Can you work these out from the model? Positions are in its coordinate system, mm. A direction names the side the tool comes from. Round coordinates to 2 decimals unless told otherwise and drop trailing zeros. Write each loop counter-clockwise with the first axis right and the second up, starting at its lowest first coordinate (ties: lowest second). Pieces come first, ordered by that corner, then holes. Notation, with made-up numbers: (40.25, 74) -> (47.25, 74) arc R15 ccw to (47.25, 100) -> close; hole circle Ø8 at (89.25, 35.25). An arc over 180 degrees is marked (long way). Use CSV: the item, a comma, the result in double quotes.
```python
from build123d import *

# Parameters (mm, degrees)
SKETCH1_W                = 29.718
SKETCH1_H                = 10.668
BOSS_EXTRUDE1_DEPTH      = 10.16
SKETCH2_W                = 10.668
SKETCH2_H                = 10.668
CUT_EXTRUDE1_DEPTH       = 7.62
M6_CLEARANCE_HOLE1_D     = 6.8032
M6_CLEARANCE_HOLE1_DEPTH = 32.4993
M6_CLEARANCE_HOLE1_TIP   = 2.043887482


with BuildPart() as part:
    # Sketch1 → Boss-Extrude1 (new body)
    with BuildSketch(Plane(origin=(0, 0, 0), x_dir=(1, 0, 0), z_dir=(0, 1, 0))):
        Rectangle(SKETCH1_W, SKETCH1_H)
    extrude(amount=BOSS_EXTRUDE1_DEPTH)

    # Sketch2 → Cut-Extrude1 (cut)
    with BuildSketch(Plane(origin=(0, 0, 0), x_dir=(-1, 0, 0), z_dir=(0, -1, 0))):
        with Locations((-9.525, 0)):
            Rectangle(SKETCH2_W, SKETCH2_H)
    extrude(amount=-CUT_EXTRUDE1_DEPTH, mode=Mode.SUBTRACT)

    # M6 Clearance Hole1
    with Locations(Plane(origin=(0, 10.16, 0), x_dir=(1, 0, 0), z_dir=(0, 1, 0))):
        with Locations((10.06602, 0)):
            Hole(M6_CLEARANCE_HOLE1_D / 2, depth=M6_CLEARANCE_HOLE1_DEPTH)
            with Locations((0, 0, -(M6_CLEARANCE_HOLE1_DEPTH + M6_CLEARANCE_HOLE1_TIP / 2))):  # 118° drill point
                Cone(0, M6_CLEARANCE_HOLE1_D / 2, M6_CLEARANCE_HOLE1_TIP, mode=Mode.SUBTRACT)


solid = part.part
```
Q1. On a 3-axis mill with a long thin cutter (end or side, diameter ignored), from which of +Z, -Z, +X, -X, +Y, -Y can I reach the whole of each face in a straight line? I mean faces 1 (the face through (-5, 0, 0)), 2 (the face through (4.191, 4, 0)). Say none if no direction works.
Resolved:
face 1,"+Z, -Z, +X, -X, -Y"
face 2,"+Z, -Z, +X, -Y"
Q2. Suppose I cut it at D-D (z = 3.75). Write out the boundary of the cut face in (x, y).
Resolved:
outline,"(-14.86, 0) -> (4.19, 0) -> (4.19, 7.62) -> (14.86, 7.62) -> (14.86, 10.16) -> (-14.86, 10.16) -> close"
Q3. Suppose I cut it at C-C (x = 12.25). Write out the boundary of the cut face in (y, z).
Resolved:
outline,"(7.62, -5.33) -> (10.16, -5.33) -> (10.16, -2.61) -> (7.62, -2.61) -> close; (7.62, 2.61) -> (10.16, 2.61) -> (10.16, 5.33) -> (7.62, 5.33) -> close"
Q4. If we mould it in two halves opening along Z, with no side actions, what happens to faces 3 (the face through (10.8, 8.87, 3.32)), 4 (the face through (7, 7.62, -2)), 5 (the face through (-4, 5, 5.334))? For each: released by +Z, released by -Z, zero draft, split by the parting line, or undercut.
Resolved:
face 3,"undercut"
face 4,"zero draft"
face 5,"released by +Z"
Q5. Will these pins go through, and if not, where does the flat tip stop? P1, Ø5, axis at x = 10.5, z = 1, coming from the -Y side; P2, Ø4, axis at y = 4.5, z = -0.5, coming from the +X side.
Resolved:
P1,"stops at y = 7.62"
P2,"stops at x = 4.19"
Q6. Please list where these lines run through material, in increasing order: probe 1 along Y at (x, z) = (6, -0.25); probe 2 along X at (y, z) = (0.75, 0); probe 3 along X at (y, z) = (9.75, -1).
Resolved:
probe 1,"y = 7.62 to 10.16"
probe 2,"x = -14.86 to 4.19"
probe 3,"x = -14.86 to 6.81, 13.32 to 14.86"
Q7. Suppose I cut it at A-A (z = 0). Write out the boundary of the cut face in (x, y).
Resolved:
outline,"(-14.86, 0) -> (4.19, 0) -> (4.19, 7.62) -> (6.66, 7.62) -> (6.66, 10.16) -> (-14.86, 10.16) -> close; (13.47, 7.62) -> (14.86, 7.62) -> (14.86, 10.16) -> (13.47, 10.16) -> close"
Q8. Suppose I cut it at B-B (y = 9.5). Write out the boundary of the cut face in (x, z).
Resolved:
outline,"(-14.86, -5.33) -> (14.86, -5.33) -> (14.86, 5.33) -> (-14.86, 5.33) -> close; hole circle Ø6.8 at (10.07, 0)"
